Read the model definition and answer for the solid it produces. Units are mm, in the model's axes. A direction names the side the tool comes from. Coordinates: 2 decimals unless noted, no trailing zeros. Use a Markdown table: item, result.
from build123d import *

# Parameters (mm, degrees)
SKETCH1_W                       = 85
SKETCH1_H                       = 70
BOSS_EXTRUDE1_DEPTH             = 6
SKETCH2_W                       = 76
SKETCH2_H                       = 61
SKETCH2_W_2                     = 65
SKETCH2_H_2                     = 52.171052632
CUT_EXTRUDE1_DEPTH              = 5
SKETCH8_W                       = 63
SKETCH8_H                       = 50
CUT_EXTRUDE2_DEPTH              = 3
SKETCH19_W                      = 85
SKETCH19_H                      = 70
SKETCH19_W_2                    = 76
SKETCH19_H_2                    = 61
CUT_EXTRUDE3_DEPTH              = 3
F_9_64_0_14063_DIAMETER_HOLE3_D = 3.572002
F_3_0MM_DOWEL_HOLE1_D           = 3
F_3_0MM_DOWEL_HOLE1_DEPTH       = 3


with BuildPart() as part:
    # Sketch1 → Boss-Extrude1 (new body)
    with BuildSketch(Plane.XY):
        Rectangle(SKETCH1_W, SKETCH1_H)
    extrude(amount=BOSS_EXTRUDE1_DEPTH)

    # Sketch2 → Cut-Extrude1 (cut)
    with BuildSketch(Plane(origin=(0, 0, 0), x_dir=(-1, 0, 0), z_dir=(0, 0, -1))):
        Rectangle(SKETCH2_W, SKETCH2_H)
        Rectangle(SKETCH2_W_2, SKETCH2_H_2, mode=Mode.SUBTRACT)
    extrude(amount=-CUT_EXTRUDE1_DEPTH, mode=Mode.SUBTRACT)

    # Sketch8 → Cut-Extrude2 (cut)
    with BuildSketch(Plane.XY.offset(6)):
        Rectangle(SKETCH8_W, SKETCH8_H)
    extrude(amount=-CUT_EXTRUDE2_DEPTH, mode=Mode.SUBTRACT)

    # Sketch19 → Cut-Extrude3 (cut)
    with BuildSketch(Plane(origin=(0, 0, 0), x_dir=(-1, 0, 0), z_dir=(0, 0, -1))):
        Rectangle(SKETCH19_W, SKETCH19_H)
        Rectangle(SKETCH19_W_2, SKETCH19_H_2, mode=Mode.SUBTRACT)
    extrude(amount=-CUT_EXTRUDE3_DEPTH, mode=Mode.SUBTRACT)

    # 9/64 (0.14063) Diameter Hole3 (through all)
    with Locations(Plane.XY.offset(3)):
        with Locations((28.529940603, -21.250215539), (28.529940603, -15.745880775), (28.529940603, -9.835912277), (28.529940603, -4.156518145), (28.529940603, 1.34781662), (28.529940603, 7.134244498), (28.529940603, 12.867155503), (28.529940603, 18.758619001), (24.333707157, 16.083468805), (24.333707157, 21.324215456), (24.333707157, 10.30729249), (24.333707157, 4.547623048), (24.333707157, -1.088505773), (24.333707157, -6.681369284), (24.333707157, -12.70462684), (24.333707157, -18.437537845), (19.848506548, -21.250215539), (19.848506548, -15.745880775), (19.848506548, -9.835912277), (19.848506548, -4.156518145), (19.848506548, 1.34781662), (19.848506548, 7.134244498), (19.848506548, 12.867155503), (19.848506548, 18.758619001), (15.547544477, 21.324215456), (15.547544477, 16.083468805), (15.547544477, 10.30729249), (15.547544477, 4.547623048), (16.308011503, -1.088505773), (15.547544477, -6.681369284), (15.547544477, -12.70462684), (15.547544477, -18.437537845), (10.648529587, -21.250215539), (10.648529587, -15.745880775), (10.648529587, -9.835912277), (10.648529587, -4.156518145), (10.648529587, 1.34781662), (10.648529587, 7.134244498), (10.648529587, 12.867155503), (10.648529587, 18.758619001), (5.705552369, 21.324215456), (5.705552369, 16.083468805), (6.382139513, 10.30729249), (5.705552369, 4.547623048), (5.705552369, -1.088505773), (5.705552369, -6.681369284), (5.705552369, -12.70462684), (5.705552369, -18.437537845), (0.781883537, -21.250215539), (0.781883537, -15.745880775), (0.781883537, -9.835912277), (0.781883537, -4.156518145), (0.781883537, 1.34781662), (0.781883537, 7.134244498), (0.781883537, 12.867155503), (0.781883537, 18.758619001), (-3.844195099, 21.324215456), (-3.844195099, 16.083468805), (-3.844195099, 10.30729249), (-3.844195099, 4.547623048), (-3.844195099, -1.088505773), (-3.844195099, -6.681369284), (-3.844195099, -12.70462684), (-3.844195099, -18.437537845), (-8.944854311, -21.250215539), (-8.944854311, -15.745880775), (-8.944854311, -9.835912277), (-8.944854311, -4.156518145), (-8.944854311, 1.34781662), (-8.944854311, 7.134244498), (-8.944854311, 12.867155503), (-8.944854311, 18.758619001), (-13.879613549, 21.324215456), (-13.879613549, 16.083468805), (-13.879613549, 10.30729249), (-13.879613549, 4.547623048), (-13.879613549, -1.088505773), (-13.879613549, -6.681369284), (-13.879613549, -12.70462684), (-13.879613549, -18.437537845), (-18.443188767, -21.250215539), (-18.443188767, -15.745880775), (-18.443188767, -9.835912277), (-18.443188767, -4.156518145), (-18.443188767, 1.34781662), (-18.443188767, 7.134244498), (-18.443188767, 12.867155503), (-18.443188767, 18.758619001), (-23.456120087, 21.324215456), (-23.456120087, 16.083468805), (-23.456120087, 10.30729249), (-23.456120087, 4.547623048), (-22.502226718, -1.088505773), (-23.456120087, -6.681369284), (-23.456120087, -12.70462684), (-23.456120087, -18.437537845), (-27.651383709, -21.250215539), (-27.651383709, -15.745880775), (-27.651383709, -9.835912277), (-27.651383709, -4.156518145), (-27.651383709, 1.34781662), (-27.651383709, 7.134244498), (-27.651383709, 12.867155503), (-27.651383709, 18.758619001)):
            Hole(F_9_64_0_14063_DIAMETER_HOLE3_D / 2)

    # Ø3.0mm Dowel Hole1
    with Locations(Plane(origin=(0, 0, 3), x_dir=(-1, 0, 0), z_dir=(0, 0, -1))):
        with Locations((13.498913812, -32.845700562), (-12.363328063, -32.845700562), (40.325591259, -22.041000365), (40.325591259, 17.495913013), (20.409683685, 32.588930896), (-27.176681905, 32.588930896), (-40.217959294, 23.331440204), (-40.217959294, -22.041000365)):
            Hole(F_3_0MM_DOWEL_HOLE1_D / 2, depth=F_3_0MM_DOWEL_HOLE1_DEPTH)


solid = part.part
(1) Straight lines are drawn through the part: L1, parallel to Y at x = -32, z = 4.4; L2, parallel to X at y = -10, z = 3.5; L3, parallel to Y at x = -18.5, z = 4.8. For each, find the intervals that lie inside material, in ascending order.
Report:
| item | result |
|---|---|
| L1 | y = -35 to -30.5, -26.09 to 26.09, 30.5 to 35 |
| L2 | x = -42.5 to -38, -32.5 to -31.5, 31.5 to 32.5, 38 to 42.5 |
| L3 | y = -35 to -30.5, -26.09 to -25, 25 to 26.09, 30.5 to 35 |
(2) Each of these flat-tipped pins is pushed along its axis until it touches: P1, Ø2.5, axis at x = 40.22, y = -22.04, coming from the -Z side; P2, Ø4, axis at x = 27, y = -13.5, coming from the +Z side. Where does it stop, or does it pass through?
Report:
| item | result |
|---|---|
| P1 | passes through |
| P2 | stops at z = 3 |
(3) A cutting plane is placed at A-A, the plane z = 4. Count the separate pieces of the cut face and the enclosed holes in it, and give its area (3 significant figures).
Report:
| item | result |
|---|---|
| separate pieces | 2 |
| enclosed holes | 10 |
| area | 1,500 mm² |
(4) The mould has two halves that part along Y. Classify faces 1 (the cylindrical face through (10.88, 20.53, 1.48)), 2 (the flat face through (42.5, 0, 4)): pulls with the +Y half, pulls with the -Y half, needs draft (parallel to the pull), parting line crosses it, or undercut.
Report:
| item | result |
|---|---|
| face 1 | undercut |
| face 2 | needs draft |
(5) For faces 3 (the flat face through (0, -25, 5)), 4 (the flat face through (0, 31, 3)), 5 (the cylindrical face through (-14.84, 17.59, 1.48)), determine the directions among +Z, -Z, +X, -X, +Y, -Y from which every point of the face is accessible in a straight line to the end or side of a thin tool.
Report:
| item | result |
|---|---|
| face 3 | +Z |
| face 4 | -Z |
| face 5 | +Z, -Z |
